from build123d import *

# Parameters (mm, degrees)
F0_W     = 21
F0_H     = 48
F0_W_2   = 52
F0_H_2   = 21
F1_DEPTH = 21
F0_W_3   = 2
F0_H_3   = 2
F2_DEPTH = 2
F3_W     = 25
F3_H     = 25
F4_DEPTH = 2
F5_W     = 25
F5_H     = 25
F6_DEPTH = 2
F7_W     = 25
F7_H     = 25
F8_DEPTH = 2
F9_R     = 2


with BuildPart() as f1:
    # F0 (on Front) → F1 (new body)
    with BuildSketch(Plane.XZ):
        with Locations((27, 36.5)):
            Rectangle(F0_W, F0_H)
        with Locations((-11.5, 0)):
            Rectangle(F0_W_2, F0_H_2)
        Polygon((14.5, -10.5), (37.5, -10.5), (37.5, 10.5), (37.5, 12.5), (16.5, 12.5), (16.5, 10.5), (14.5, 10.5), align=None)
    extrude(amount=F1_DEPTH)

    # F0 (on Front) → F2 (join)
    with BuildSketch(Plane.XZ):
        Polygon((37.5, 10.5), (37.5, -10.5), (14.5, -10.5), (14.5, -12.5), (39.5, -12.5), (39.5, 12.5), (37.5, 12.5), align=None)
        with Locations((15.5, 11.5)):
            Rectangle(F0_W_3, F0_H_3)
        Polygon((14.5, -10.5), (37.5, -10.5), (37.5, 10.5), (37.5, 12.5), (16.5, 12.5), (16.5, 10.5), (14.5, 10.5), align=None)
    extrude(amount=-F2_DEPTH)

    # F3 (on face) → F4 (join)
    with BuildSketch(Plane.XZ.offset(21)):
        with Locations((27, 0)):
            Rectangle(F3_W, F3_H)
    extrude(amount=F4_DEPTH)

    # F5 (on face) → F6 (join)
    with BuildSketch(Plane.YZ.offset(37.5)):
        with Locations((-10.5, 0)):
            Rectangle(F5_W, F5_H)
    extrude(amount=F6_DEPTH)

    # F7 (on face) → F8 (join)
    with BuildSketch(Plane(origin=(0, 0, -10.5), x_dir=(1, 0, 0), z_dir=(0, 0, -1))):
        with Locations((27, 10.5)):
            Rectangle(F7_W, F7_H)
    extrude(amount=F8_DEPTH)

    # F9
    f9_edges = [f1.edges().sort_by_distance(p)[0] for p in [
        (-37.5, -10.5, -10.5),
        (-37.5, 0, 0),
        (-37.5, -10.5, 10.5),
        (-37.5, -21, 0),
        (27, 0, 60.5),
        (16.5, -10.5, 60.5),
        (37.5, -10.5, 60.5),
        (27, -21, 60.5),
        (16.5, -21, 36.5),
        (37.5, -21, 36.5),
        (37.5, 0, 36.5),
        (16.5, 0, 36.5),
        (-11.5, 0, 10.5),
        (-11.5, 0, -10.5),
        (-11.5, -21, 10.5),
        (-11.5, -21, -10.5),
    ]]
    fillet(f9_edges, radius=F9_R)


solid = f1.part
Check sheet for the modelled part. Datum: model origin and axes. Units: mm. A direction names the side the tool comes from. Coordinates: 2 decimals unless noted, no trailing zeros. Write each loop counter-clockwise with the first axis right and the second up, starting at its lowest first coordinate (ties: lowest second). Pieces come first, ordered by that corner, then holes.
Item 1: Cross-section at A-A on x = 2. Record the boundary of the cut face in (y, z).
Numbers:
outline: (-21, -8.5) arc R2 ccw to (-19, -10.5) - (-2, -10.5) arc R2 ccw to (0, -8.5) - (0, 8.5) arc R2 ccw to (-2, 10.5) - (-19, 10.5) arc R2 ccw to (-21, 8.5) - close
Item 2: Cross-section at C-C on y = -18. Record the boundary of the cut face in (x, z), then the cut area to 3 significant figures.
Numbers:
outline: (-37.5, -8.5) arc R2 ccw to (-35.5, -10.5) - (14.5, -10.5) - (14.5, -12.5) - (39.5, -12.5) - (39.5, 12.5) - (37.5, 12.5) - (37.5, 58.5) arc R2 ccw to (35.5, 60.5) - (18.5, 60.5) arc R2 ccw to (16.5, 58.5) - (16.5, 10.5) - (-35.5, 10.5) arc R2 ccw to (-37.5, 8.5) - close
area: 2,720 mm2
Item 3: Mould release check, pull along Y, two halves, no side actions. Record for faces 6 (the face through (15, 0, 12)), 7 (the face through (15, -21, 12)), 8 (the face through (39.5, -10, 0)), 9 (the face through (27.12, -0.6, 59.93)): released by +Y, released by -Y, zero draft, split by the parting line, or undercut.
Numbers:
face 6: undercut
face 7: undercut
face 8: zero draft
face 9: released by +Y
Item 4: Scan lines: probe 1 along Y at (x, z) = (23.5, 18.5); probe 2 along Z at (x, y) = (11.5, -10); probe 3 along Z at (x, y) = (33, -21.5). Record each from-to range of solid material in increasing order.
Numbers:
probe 1: y = -21 to 0
probe 2: z = -10.5 to 10.5
probe 3: z = -12.5 to 12.5
Item 5: Access from +Z, -Z, +X, -X, +Y, -Y to the whole of each face (thin tool, end or side, straight path). Record for faces 1 (the face through (-11, -21, 0)), 2 (the face through (-10.85, -0.6, 9.93)), 3 (the face through (37.5, -10, 35)), 4 (the face through (27, -21, 36)), 5 (the face through (-10.15, -0.6, -9.93)).
Numbers:
face 1: +Z, -Z, -X, -Y
face 2: +Z, -X, +Y
face 3: +Z, +X, +Y, -Y
face 4: +Z, +X, -X, -Y
face 5: -Z, -X, +Y
Item 6: Cross-section at B-B on z = 31. Record the boundary of the cut face in (x, y), then the cut area to 3 significant figures.
Numbers:
outline: (16.5, -19) arc R2 ccw to (18.5, -21) - (35.5, -21) arc R2 ccw to (37.5, -19) - (37.5, -2) arc R2 ccw to (35.5, 0) - (18.5, 0) arc R2 ccw to (16.5, -2) - close
area: 438 mm2
Item 7: Depth check by flat-ended pin: pin 1 Ø13.5 at (x, z) = (30, 35.5) entering from -Y; pin 2 Ø13.5 at (x, z) = (-11, -0.5) entering from +Y; pin 3 Ø8 at (x, z) = (13.5, 29) entering from -Y. Enter the tip coordinate at first touch or a pass-through.
Numbers:
pin 1: stops at y = -21
pin 2: stops at y = 0
pin 3: stops at y = -20.73
Item 8: Cross-section at D-D on x = 25.5. Record the boundary of the cut face in (y, z), then the cut area to 3 significant figures.
Numbers:
outline: (-23, -12.5) - (2, -12.5) - (2, 12.5) - (0, 12.5) - (0, 58.5) arc R2 ccw to (-2, 60.5) - (-19, 60.5) arc R2 ccw to (-21, 58.5) - (-21, 12.5) - (-23, 12.5) - close
area: 1,630 mm2
